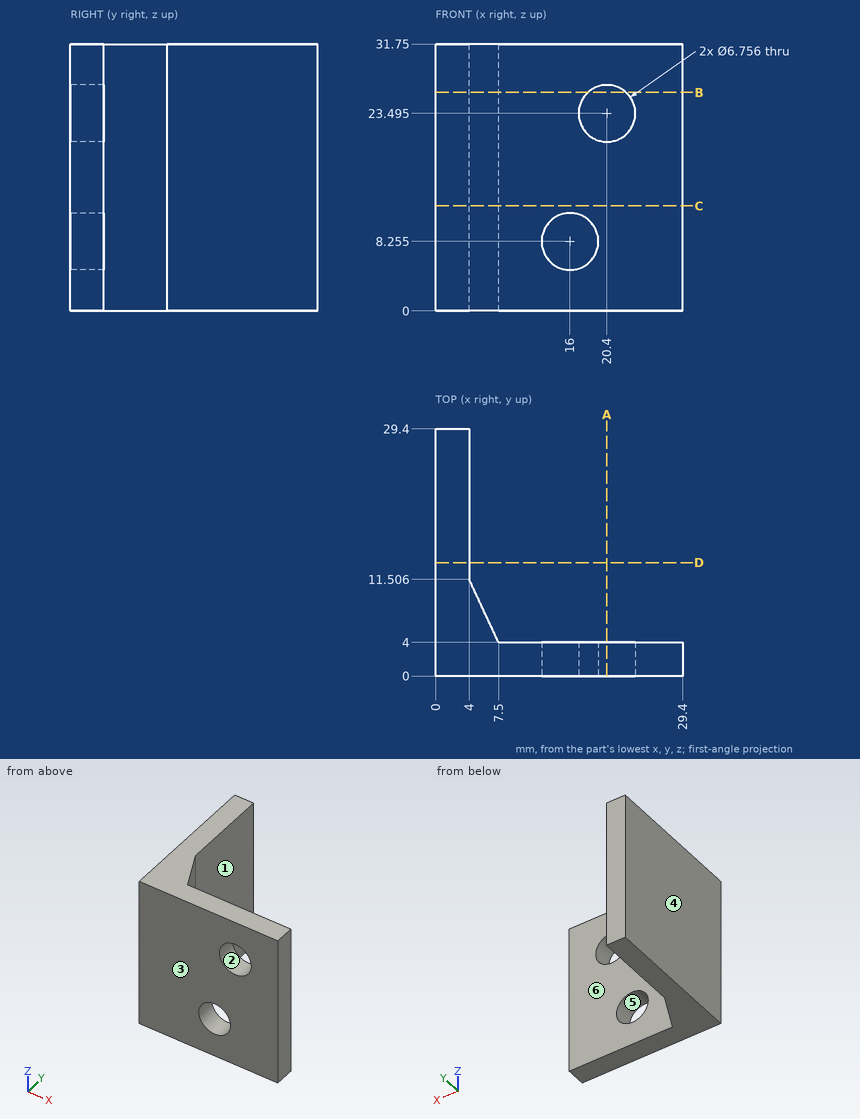
Geometry: see drawing. Coordinates: mm, zero at the bounding-box minimum. A direction names the side the tool comes from. Round coordinates to 2 decimals unless told otherwise and drop trailing zeros. Write each loop counter-clockwise with the first axis right and the second up, starting at its lowest first coordinate (ties: lowest second). Pieces come first, ordered by that corner, then holes.
1) Contact query for flat-ended pins moving along their axis: P1, Ø1.5, axis at x = 5, z = 21.5, coming from the -Y side; P2, Ø10, axis at y = 17.5, z = 24.5, coming from the +X side; P3, Ø6.5, axis at x = 15.5, z = 11.5, coming from the +Y side. Output: stop coordinate, or through.
2) Cut plane B-B (z = 26). Return the cut outline in (x, y) (1 decimal).
3) Cut plane D-D (y = 13.5). Return the cut outline in (x, z).
4) Ray query, L1, parallel to Z at x = 16, y = 1.1; L2, parallel to Z at x = 20.4, y = 0.9; L3, parallel to X at y = 14.5, z = 20. Return the intervals inside material, ascending.
5) Reachability of the marked faces 5 and 6 from +Z, -Z, +X, -X, +Y, -Y: full face, straight path, thin tool, end or side. Return the list, or none.
6) Cut plane C-C (z = 12.5). Return the cut outline in (x, y) (1 decimal).
7) Cut plane A-A (x = 20.4). Return the cut outline in (y, z).
8) Draft query along X for the marked faces 1, 2, 3 and 4. Return one class per face: pulls with the +X half, pulls with the -X half, needs draft (parallel to the pull), parting line crosses it, or undercut.
Geometry says:
1. P1: stops at y = 0
1. P2: stops at x = 4
1. P3: stops at y = 4
2. outline: (0, 0) - (18.1, 0) - (18.1, 4) - (7.5, 4) - (4, 11.5) - (4, 29.4) - (0, 29.4) - close; (22.7, 0) - (29.4, 0) - (29.4, 4) - (22.7, 4) - close
3. outline: (0, 0) - (4, 0) - (4, 31.75) - (0, 31.75) - close
4. L1: z = 0 to 4.88, 11.63 to 31.75
4. L2: z = 0 to 20.12, 26.87 to 31.75
4. L3: x = 0 to 4
5. face 5: +Y, -Y
5. face 6: +Z, -Z, +X, +Y
6. outline: (0, 0) - (29.4, 0) - (29.4, 4) - (7.5, 4) - (4, 11.5) - (4, 29.4) - (0, 29.4) - close
7. outline: (0, 0) - (4, 0) - (4, 20.12) - (0, 20.12) - close; (0, 26.87) - (4, 26.87) - (4, 31.75) - (0, 31.75) - close
8. face 1: pulls with the +X half
8. face 2: undercut
8. face 3: needs draft
8. face 4: pulls with the -X half
